Geometry: final body of the model. Coordinates: model frame, mm. A direction names the side the tool comes from. Coordinates: 2 decimals unless noted, no trailing zeros. Order: outer loops, then holes, each group sorted by start corner. A loop starts at its lowest first (then second) coordinate and runs counter-clockwise, first axis right, second up. Notation, with made-up numbers: (-12.5, 8.5) -> (1.5, 8.5) arc R14 ccw to (1.5, 12.5) -> close; hole circle Ø2 at (88.25, 22.5). An arc over 180 degrees is marked (long way). Use CSV: the item, a comma, the result in double quotes. Start each with the question number.
from build123d import *

# Parameters (mm, degrees)
F0_W     = 116.462328
F0_H     = 72.291564
F0_R     = 1.5
F0_W_2   = 108.797777
F0_H_2   = 64.347155
F1_DEPTH = 3


with BuildPart() as f1:
    # F0 (on Top) → F1 (new body)
    with BuildSketch(Plane.XY):
        with Locations((0.074979, -0.045983)):
            Rectangle(F0_W, F0_H)
        with Locations((-56.5, -33.5)):
            Circle(F0_R, mode=Mode.SUBTRACT)
        with Locations((56.5, -33.5)):
            Circle(F0_R, mode=Mode.SUBTRACT)
        with Locations((0.575187, -0.244237)):
            Rectangle(F0_W_2, F0_H_2, mode=Mode.SUBTRACT)
        with Locations((-56.5, 33.5)):
            Circle(F0_R, mode=Mode.SUBTRACT)
        with Locations((56.5, 33.5)):
            Circle(F0_R, mode=Mode.SUBTRACT)
    extrude(amount=F1_DEPTH)


solid = f1.part
(1) Line query: line 1 (Y direction, x = -56.5, z = 1.5); line 2 (X direction, y = 25, z = 1.4); line 3 (Y direction, x = -39, z = 2.85). Output: solid intervals per line, ascending. Write a range as from..to.
(2) First-contact query: pin 1 (2.5 mm diameter, centred on x = 56.5, y = -33.5, fed in from -Z). Flat tip, straight axial feed; report the tip coordinate or a pass-through.
(3) Section C-C (x = -27.5). Return loops of the section in (y, z), then the cut area to 3 significant figures.
(4) Section A-A (x = -56.5). Return loops of the section in (y, z), then the cut area to 3 significant figures.
(5) Section B-B (y = 16.5). Return loops of the section in (x, z).
(6) Section D-D (z = 1.15). Return loops of the section in (x, y), then the cut area to 3 significant figures.
(7) Access query for faces 4 (the face through (0, 31.929, 1)), 5 (the face through (-1, -36.192, 1)). Directions: +Z, -Z, +X, -X, +Y, -Y. A direction counts if a zero-diameter tool reaches every point of the face in a straight line with its end or side. Return the directions, or none.
(8) Mould query, pull axis X, two halves, no side actions, for faces 1 (the face through (-4.5, 32.3, 0)), 2 (the face through (58.306, -1, 1)), 3 (the face through (57.886, 32.925, 1.479)). Classes: pulls with the +X half, pulls with the -X half, needs draft (parallel to the pull), parting line crosses it, or undercut.
Check sheet entries:
1,line 1,"y = -36.19..-35, -32..32, 35..36.1"
1,line 2,"x = -58.16..-53.82, 54.97..58.31"
1,line 3,"y = -36.19..-32.42, 31.93..36.1"
2,pin 1,"passes through"
3,outline,"(-36.19, 0) -> (-32.42, 0) -> (-32.42, 3) -> (-36.19, 3) -> close; (31.93, 0) -> (36.1, 0) -> (36.1, 3) -> (31.93, 3) -> close"
3,area,"23.8 mm^2"
4,outline,"(-36.19, 0) -> (-35, 0) -> (-35, 3) -> (-36.19, 3) -> close; (-32, 0) -> (32, 0) -> (32, 3) -> (-32, 3) -> close; (35, 0) -> (36.1, 0) -> (36.1, 3) -> (35, 3) -> close"
4,area,"199 mm^2"
5,outline,"(-58.16, 0) -> (-53.82, 0) -> (-53.82, 3) -> (-58.16, 3) -> close; (54.97, 0) -> (58.31, 0) -> (58.31, 3) -> (54.97, 3) -> close"
6,outline,"(-58.16, -36.19) -> (58.31, -36.19) -> (58.31, 36.1) -> (-58.16, 36.1) -> close; hole circle Ø3 at (-56.5, -33.5); hole circle Ø3 at (-56.5, 33.5); hole (-53.82, -32.42) -> (54.97, -32.42) -> (54.97, 31.93) -> (-53.82, 31.93) -> close; hole circle Ø3 at (56.5, -33.5); hole circle Ø3 at (56.5, 33.5)"
6,area,"1,390 mm^2"
7,face 4,"+Z, -Z"
7,face 5,"+Z, -Z, +X, -X, -Y"
8,face 1,"needs draft"
8,face 2,"pulls with the +X half"
8,face 3,"undercut"
